For this review, take the finished solid that the model builds, in its own axes (mm). A direction names the side the tool comes from. Round coordinates to 2 decimals unless told otherwise and drop trailing zeros. Write each question's results on one line, items separated by ' | '. Start each with the question number.
(1) For faces 1 (the flat face through (0, 22, 2)), 2 (the flat face through (115, 5, 2)), list the 3-axis set-ups (+Z, -Z, +X, -X, +Y, -Y) from which the entire face can be reached by the end or side of a thin tool; tool diameter is ignored.
(2) For L1, parallel to Y at x = 227.5, z = 3.3; L2, parallel to X at y = 3.5, z = 4.1, list the stretches that pass through material, from the lowest coordinate up. Write a range as from..to.
(3) Insertion check: pin 1 Ø8 at (x, y) = (142.5, 13.5) entering from -Z; pin 2 Ø1.5 at (x, z) = (115, 2.5) entering from -Y. Each pin has a flat end and moves straight along its axis. Give the tip position at first contact, or say it passes through.
```python
from build123d import *

# Parameters (mm, degrees)
SKETCH1_W           = 230
SKETCH1_H           = 45
BOSS_EXTRUDE1_DEPTH = 5
SKETCH2_R           = 1.5
CUT_EXTRUDE1_DEPTH  = 10
SKETCH3_W           = 15.24
SKETCH3_H           = 10
CUT_EXTRUDE2_DEPTH  = 5


with BuildPart() as part:
    # Sketch1 → Boss-Extrude1 (new body)
    with BuildSketch(Plane.XY):
        with Locations((115, 22.5)):
            Rectangle(SKETCH1_W, SKETCH1_H)
    extrude(amount=BOSS_EXTRUDE1_DEPTH)

    # Sketch2 → Cut-Extrude1 (cut)
    with BuildSketch(Plane(origin=(0, 0, 0), x_dir=(-1, 0, 0), z_dir=(0, 0, -1))):
        with Locations((-227.5, 42.5)):
            Circle(SKETCH2_R)
        with Locations((-227.5, 2.5)):
            Circle(SKETCH2_R)
        with Locations((-2.5, 2.5)):
            Circle(SKETCH2_R)
        with Locations((-2.5, 42.5)):
            Circle(SKETCH2_R)
    extrude(amount=-CUT_EXTRUDE1_DEPTH, mode=Mode.SUBTRACT)

    # Sketch3 → Cut-Extrude2 (cut)
    with BuildSketch(Plane(origin=(0, 0, 0), x_dir=(-1, 0, 0), z_dir=(0, 0, -1))):
        with Locations((-115, 0)):
            Rectangle(SKETCH3_W, SKETCH3_H)
    extrude(amount=-CUT_EXTRUDE2_DEPTH, mode=Mode.SUBTRACT)


solid = part.part
```
Results below:
1) face 1: +Z, -Z, -X, +Y, -Y | face 2: +Z, -Z, -Y
2) L1: y = 0..1, 4..41, 44..45 | L2: x = 0..1.38, 3.62..107.38, 122.62..226.38, 228.62..230
3) pin 1: stops at z = 0 | pin 2: stops at y = 5
